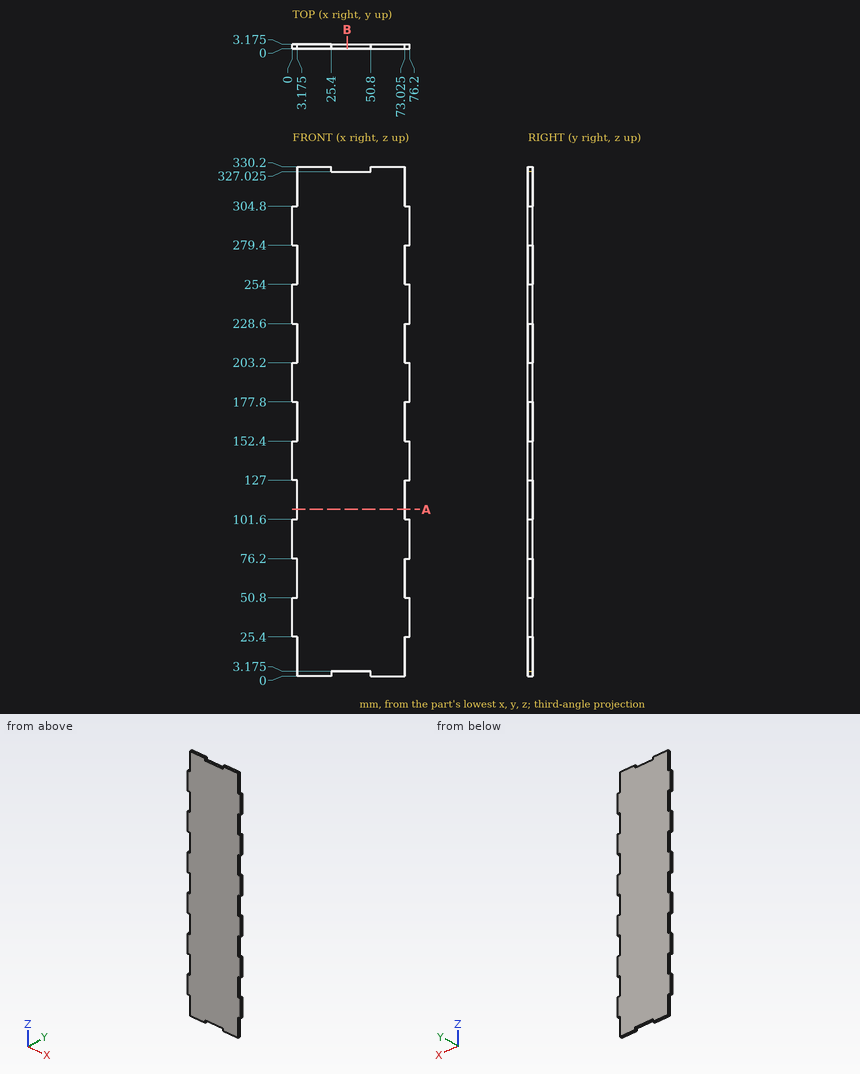
The figure shows three views and two pictorial views of one solid part (mm, origin at its lowest corner). Answer the questions. Coordinates: 2 decimals unless noted, no trailing zeros. Order: outer loops, then holes, each group sorted by start corner. A loop starts at its lowest first (then second) coordinate and runs counter-clockwise, first axis right, second up. Notation, with made-up numbers: (-2, 72.5) - (53, 72.5) arc R13 cw to (53, 96.5) - close; hole circle Ø10 at (86.25, 50). An arc over 180 degrees is marked (long way). Answer as a JSON object with one key per item and string values.
1. Each of these flat-tipped pins is pushed along its axis until it touches: P1, Ø1.6, axis at x = 1, y = 2, coming from the -Z side; P2, Ø1.6, axis at x = 74.5, y = 1.5, coming from the +Z side; P3, Ø1.6, axis at y = 2, z = 323, coming from the +X side (3 decimals). Where does it stop, or does it pass through?
Output values:
{"P1": "stops at z = 25.4", "P2": "stops at z = 304.8", "P3": "stops at x = 73.025"}
2. Consider line 1 (Z direction, x = 28, y = 1.3) (3 decimals); line 2 (X direction, y = 2.25, z = 310.5) (3 decimals). Determine where each line is inside the solid, lowest interval first.
Output values:
{"line 1": "z = 3.175 to 327.025", "line 2": "x = 3.175 to 73.025"}
3. Find section B-B on x = 35.5. Determine the outline of the cut face in (y, z) (3 decimals), plus the area to 3 significant figures.
Output values:
{"outline": "(0, 3.175) - (3.175, 3.175) - (3.175, 327.025) - (0, 327.025) - close", "area": "1,030 mm²"}
4. Find section A-A on z = 108. Determine the outline of the cut face in (x, y) (3 decimals), plus the area to 3 significant figures.
Output values:
{"outline": "(3.175, 0) - (73.025, 0) - (73.025, 3.175) - (3.175, 3.175) - close", "area": "222 mm²"}
